from build123d import *

# Parameters (mm, degrees)
F1_DEPTH = 46.25


with BuildPart() as f1:
    # F0 (on Front) → F1 (new body)
    with BuildSketch(Plane.XZ):
        with BuildLine():
            ThreePointArc((38.958571, 29.182484), (30.880263, 33.122538), (32.748961, 24.331006))
            ThreePointArc((32.748961, 24.331006), (37.036878, 25.242431), (38.958571, 29.182484))
        make_face()
        with BuildLine():
            ThreePointArc((16.559277, -8.999688), (16.643621, -10.295744), (16.895229, -11.569936))
            ThreePointArc((16.895229, -11.569936), (20.464299, -16.927566), (26.559277, -18.999688))
            Line((26.559277, -18.999688), (41.197145, -18.999688))
            Line((41.197145, -18.999688), (41.197145, 6.000312))
            Line((41.197145, 6.000312), (41.197145, 13.000312))
            Line((41.197145, 13.000312), (41.197145, 26.612237))
            ThreePointArc((41.197145, 26.612237), (38.268212, 33.683304), (31.197145, 36.612237))
            Line((31.197145, 36.612237), (26.559277, 36.612237))
            ThreePointArc((26.559277, 36.612237), (19.488209, 33.683304), (16.559277, 26.612237))
            Line((16.559277, 26.612237), (16.559277, -8.999688))
        make_face()
        with BuildLine():
            ThreePointArc((28.797851, -11.569936), (23.797851, -16.569936), (18.797851, -11.569936))
            ThreePointArc((18.797851, -11.569936), (20.719544, -7.629882), (25.00746, -6.718458))
            ThreePointArc((25.00746, -6.718458), (27.737905, -8.491629), (28.797851, -11.569936))
        make_face(mode=Mode.SUBTRACT)
        with BuildLine():
            ThreePointArc((38.958571, 29.182484), (37.036878, 25.242431), (32.748961, 24.331006))
            ThreePointArc((32.748961, 24.331006), (30.880263, 33.122538), (38.958571, 29.182484))
        make_face(mode=Mode.SUBTRACT)
    extrude(amount=F1_DEPTH)


solid = f1.part
Geometry check sheet. Reference: the model listing, model coordinates, mm. Round coordinates to 2 decimals unless told otherwise and drop trailing zeros. Order: outer loops, then holes, each group sorted by start corner. A loop starts at its lowest first (then second) coordinate and runs counter-clockwise, first axis right, second up. Notation, with made-up numbers: (45.25, 47) - (96.25, 47) arc R21 cw to (96.25, 72) - close; hole circle Ø9 at (-17, 48). An arc over 180 degrees is marked (long way). One line per question, with ' | ' between items. Start each with the question number.
(1) Sectioned sample at A-A on y = -12.5. Record the cut outline in (x, z), and give its area (3 significant figures).
(2) Sectioned sample at C-C on z = 25.5. Record the cut outline in (x, y), and give its area (3 significant figures).
(3) Thickness scan on L1, parallel to Z at x = 23.25, y = -27.5; L2, parallel to Z at x = 26.5, y = -24; L3, parallel to X at y = -31, z = -12. Record the ranges inside material, lowest first. Write a range as [from, to].
(4) Depth check by flat-ended pin: pin 1 Ø1 at (x, z) = (35, 25.5) entering from +Y. Enter the tip coordinate at first touch or a pass-through.
(5) Sectioned sample at B-B on x = 37. Record the cut outline in (y, z).
Conclusion:
1) outline: (16.56, -9) arc R10 ccw to (16.9, -11.57) arc R10 ccw to (26.56, -19) - (41.2, -19) - (41.2, 26.61) arc R10 ccw to (31.2, 36.61) - (26.56, 36.61) arc R10 ccw to (16.56, 26.61) - close; hole (25.01, -6.72) arc R5 ccw (long way) to (28.8, -11.57) arc R5 ccw to start; hole circle Ø10 at (33.96, 29.18) | area: 1,150 mm2
2) outline: (16.56, -46.25) - (30.58, -46.25) - (30.58, 0) - (16.56, 0) - close; (37.34, -46.25) - (41.2, -46.25) - (41.2, 0) - (37.34, 0) - close | area: 827 mm2
3) L1: z = [-18.44, -16.54], [-6.6, 36.05] | L2: z = [-19, -15.78], [-7.36, 36.61] | L3: x = [17.02, 18.82], [28.78, 41.2]
4) pin 1: passes through
5) outline: (-46.25, -19) - (0, -19) - (0, 25.21) - (-46.25, 25.21) - close; (-46.25, 33.15) - (0, 33.15) - (0, 34.76) - (-46.25, 34.76) - close
